For this review, take the finished solid that the model builds, in its own axes (mm). A direction names the side the tool comes from. Coordinates: 2 decimals unless noted, no trailing zeros. Loops run counter-clockwise (first coordinate to the right, second up) from the corner with the lowest first, then second, coordinate; pieces in that order, holes last. Notation, with made-up numbers: (-22.5, 44.5) - (19.5, 44.5) arc R17 ccw to (19.5, 52.5) - close; hole circle Ø5 at (-21, 17). An arc over 180 degrees is marked (long way). Answer as a JSON object with one key per item and string values. Group by question number.
Item 1: We need section B-B (y = -52.5). Give the boundary of the cut face in (x, z) (3 decimals), then the cut area to 3 significant figures.
Item 2: To check wall thickness, follow line 1 (X direction, y = -21.5, z = 6) (3 decimals); line 2 (X direction, y = -10, z = 14) (3 decimals); line 3 (Z direction, x = -16, y = -28) (3 decimals). State the ranges of each line that lie inside material, in increasing order.
Item 3: Clearance check with flat-ended pins moving along their axes: pin 1 (6 mm diameter, centred on x = 41, z = 50, fed in from +Y); pin 2 (12 mm diameter, centred on x = 5, z = 17, fed in from -Y); pin 3 (5 mm diameter, centred on y = -13, z = 39, fed in from +X). State where each tip first meets the part, or that it passes through.
Item 4: We need section A-A (z = 4). Give the boundary of the cut face in (x, y) (3 decimals), then the cut area to 3 significant figures.
Item 5: Tool access review of faces 1 (the conical face through (109.2, -9.68, 55.78)), 2 (the cylindrical face through (45.8, -0.4, 38.1)), 3 (the flat face through (7, 7.938, 34)), 4 (the flat face through (22.225, -17, 18)), 5 (the flat face through (41.275, -1, 4)): name each direction out of +Z, -Z, +X, -X, +Y, -Y from which nothing blocks a thin tool from reaching the whole face with its end or side.
from build123d import *

# Parameters (mm, degrees)
F1_DEPTH = 63.5
F2_DEPTH = 25.4
F3_DEPTH = 7.9375
F5_R     = 5.08


with BuildPart() as f1:
    # F0 (on Front) → F1 (new body, symmetric)
    with BuildSketch(Plane.XZ):
        Polygon((41.275, -9.525), (41.275, 9.525), (22.225, 9.525), (-41.275, 9.525), (-41.275, -9.525), align=None)
    extrude(amount=F1_DEPTH, both=True)

    # F0 (on Front) → F2 (join, symmetric)
    with BuildSketch(Plane.XZ):
        with BuildLine():
            Line((22.225, 9.525), (41.275, 9.525))
            Line((41.275, 9.525), (41.275, 27.0002))
            ThreePointArc((41.275, 27.0002), (45.9246798487, 38.2255201513), (57.15, 42.8752))
            Line((57.15, 42.8752), (60.325, 42.8752))
            Line((60.325, 42.8752), (60.325, 61.9252))
            Line((60.325, 61.9252), (57.15, 61.9252))
            ThreePointArc((57.15, 61.9252), (32.4542956671, 51.6959043329), (22.225, 27.0002))
            Line((22.225, 27.0002), (22.225, 9.525))
        make_face()
        Polygon((60.325, 61.9252), (60.325, 42.8752), (60.325, 38.1), (85.725, 38.1), (85.8855976067, 61.9252), align=None)
    extrude(amount=F2_DEPTH, both=True)

    # F0 (on Front) → F3 (join, symmetric)
    with BuildSketch(Plane.XZ):
        with BuildLine():
            Line((-41.275, 9.525), (22.225, 9.525))
            Line((22.225, 9.525), (22.225, 27.0002))
            ThreePointArc((22.225, 27.0002), (32.4542956671, 51.6959043329), (57.15, 61.9252))
            add(Edge.make_bspline(
                [(-41.275, 9.525), (-11.5636568516, 48.5677458346), (20.2601272613, 70.6769004464), (57.15, 61.9252)],
                knots=[0, 0, 0, 0, 111.5045361635, 111.5045361635, 111.5045361635, 111.5045361635], degree=3))
        make_face()
    extrude(amount=F3_DEPTH, both=True)

    # F0 (on Front) → F4 (revolve)
    with BuildSketch(Plane.XZ):
        Polygon((85.9176144004, 66.675), (85.8855976067, 61.9252), (85.725, 38.1), (111.125, 38.1), (111.125, 66.675), align=None)
    revolve(axis=Axis((85.8213072002, 0, 52.3875), (0.0067405083, 0, 0.9999772825)))

    # F5
    f5_edges = [f1.edges().sort_by_distance(p)[0] for p in [
        (41.275, -63.5, 0),
        (-41.275, -63.5, 0),
        (41.275, 63.5, 0),
        (-41.275, 63.5, 0),
    ]]
    fillet(f5_edges, radius=F5_R)


solid = f1.part
Check sheet entries:
{
 "1": {"outline": "(-41.275, -9.525) - (41.275, -9.525) - (41.275, 9.525) - (-41.275, 9.525) - close", "area": "1,570 mm2"},
 "2": {"line 1": "x = -41.275 to 41.275", "line 2": "x = 22.225 to 41.275", "line 3": "z = -9.525 to 9.525"},
 "3": {"pin 1": "stops at y = 25.4", "pin 2": "stops at y = -7.94", "pin 3": "stops at x = 108.85"},
 "4": {"outline": "(-41.275, -58.42) arc R5.08 ccw to (-36.195, -63.5) - (36.195, -63.5) arc R5.08 ccw to (41.275, -58.42) - (41.275, 58.42) arc R5.08 ccw to (36.195, 63.5) - (-36.195, 63.5) arc R5.08 ccw to (-41.275, 58.42) - close", "area": "10,500 mm2"},
 "5": {"face 1": "+Z", "face 2": "-Z, +Y, -Y", "face 3": "+Z, -X, +Y", "face 4": "+Z, -X, -Y", "face 5": "-Z, +X, +Y, -Y"}
}
